Geometry check sheet. Reference: the model listing, model coordinates, mm. Give positions to 0.01 mm unless a question says otherwise; leave off trailing zeros. Order: outer loops, then holes, each group sorted by start corner. A loop starts at its lowest first (then second) coordinate and runs counter-clockwise, first axis right, second up. Notation, with made-up numbers: M -36.75,87.5 L 1.25,87.5 A19 ccw 1.25,109.5 Z; hole C -30.5,30.5 d11. An arc over 180 degrees is marked long. Use CSV: the item, a comma, the result in double quotes. Start each with the question number.
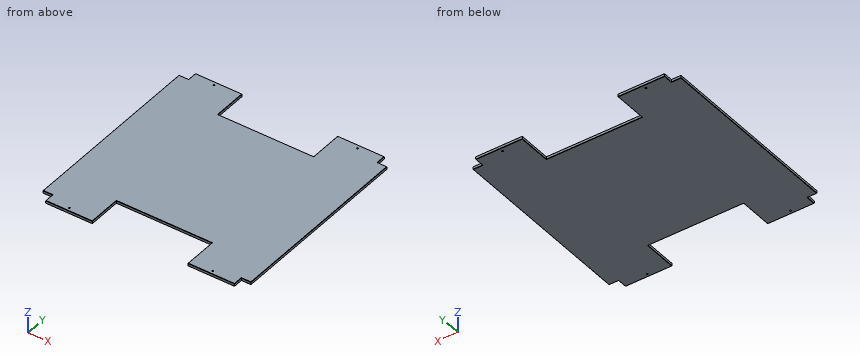
Autodesk Inventor part; units mm, degrees
ref_plane "YZ Plane" through (0, 0, 0) normal (1, 0, 0) x (0, 1, 0)
ref_plane "XZ Plane" through (0, 0, 0) normal (0, 1, 0) x (-1, 0, 0)
ref_plane "XY Plane" through (0, 0, 0) normal (0, 0, 1) x (1, 0, 0)
sketch "Skizze1" plane through (0, 0, 0) normal (0, 0, 1) x (1, 0, 0)
  line L0 (0, 0) -> (0, 395)
  line L1 (0, 395) -> (-20, 395)
  line L2 (-20, 395) -> (-20, 415)
  line L3 (-20, 415) -> (-117.5, 415)
  line L4 (-117.5, 415) -> (-117.5, 345)
  line L5 (-117.5, 345) -> (-317.5, 345)
  line L6 (-317.5, 345) -> (-317.5, 415)
  line L7 (-317.5, 415) -> (-415, 415)
  line L8 (-415, 415) -> (-415, 395)
  line L9 (-415, 395) -> (-435, 395)
  line L10 (-435, 395) -> (-435, 0)
  line L11 (-435, 0) -> (-415, 0)
  line L12 (-415, 0) -> (-415, -20)
  line L13 (-415, 0) -> (-395, 0) construction
  line L14 (-415, -20) -> (-317.5, -20)
  line L15 (-317.5, -20) -> (-317.5, 50)
  line L16 (-317.5, 50) -> (-117.5, 50)
  line L17 (-117.5, 50) -> (-117.5, -20)
  line L18 (-117.5, -20) -> (-20, -20)
  line L19 (-20, -20) -> (-20, 0)
  line L20 (-20, 0) -> (0, 0)
  dimension "d0" = 395
  dimension "d1" = 20
  dimension "d2" = 20
  dimension "d3" = 97.5
  dimension "d4" = 90
  dimension "d5" = 70
  dimension "d6" = 90
  dimension "d7" = 200
  dimension "d8" = 70
  dimension "d9" = 90
  dimension "d10" = 97.5
  dimension "d11" = 20
  dimension "d12" = 90
  dimension "d13" = 20
  dimension "d14" = 90
  dimension "d15" = 395
  dimension "d16" = 90
  dimension "d17" = 20
  dimension "d18" = 20
  dimension "d19" = 90
  dimension "d20" = 70
  dimension "d21" = 90
extrude "Extrusion1" add sketch "Skizze1" along normal blind 6
chamfer "Fase1" distance 0.5 angle 45 40 edges at (0, 197.5, 6) (-10, 0, 6) (-20, -10, 6) (-68.75, -20, 6) (-117.5, 15, 6) (-217.5, 50, 6) (-317.5, 15, 6) (-366.25, -20, 6) (-415, -10, 6) (-425, 0, 6) (-435, 197.5, 6) (-425, 395, 6) (-366.25, 415, 6) (-415, 405, 6) (-317.5, 380, 6) (-217.5, 345, 6) (-117.5, 380, 6) (-68.75, 415, 6) (-20, 405, 6) (-10, 395, 6) (-425, 0, 0) (-415, -10, 0) (-435, 197.5, 0) (-366.25, -20, 0) (-217.5, 50, 0) (-317.5, 15, 0) (-117.5, 15, 0) (-68.75, -20, 0) (-20, -10, 0) (-10, 0, 0) (0, 197.5, 0) (-10, 395, 0) (-20, 405, 0) (-68.75, 415, 0) (-117.5, 380, 0) (-217.5, 345, 0) (-317.5, 380, 0) (-425, 395, 0) (-415, 405, 0) (-366.25, 415, 0)
sketch "Skizze2" plane through (0, 0, 6) normal (0, 0, 1) x (1, 0, 0)
  circle A0 centre (-70.5, 407) radius 1.6
  line L0 (-117, 414.5) -> (-20.5, 414.5)
  line L1 (-20.5, 414.5) -> (-20.5, 394.5)
  circle A1 centre (-370.5, 407) radius 1.6
  circle A2 centre (-70.5, -13) radius 1.6
  circle A3 centre (-370.5, -13) radius 1.6
  point P0 (0, 0)
  dimension "d27" = 3.2
  dimension "d28" = 7.5
  dimension "d29" = 50
  dimension "d32" = 300
  dimension "d35" = 420
extrude "Extrusion2" cut sketch "Skizze2" against normal through all
properties part number "middle plate" material "Birke"
(1) Sectioned sample at C-C on x = -270. Record the cut outline in (y, z).
(2) Sectioned sample at A-A on z = 1.75. Record the cut outline in (x, y), then the cut area to 3 significant figures.
(3) Go/stop test with flat-tipped pins: P1, Ø3.5, axis at x = -70.5, y = -13, coming from the -Z side; P2, Ø2.5, axis at y = 408.5, z = 3.5, coming from the -X side; P3, Ø2.5, axis at x = -10, z = 3, coming from the -Y side; P4, Ø1.5, axis at x = -5.5, z = 3, coming from the +Y side. Record where each tip stops, or that it passes through.
(4) Sectioned sample at B-B on y = 19.5. Record the cut outline in (x, z), then the cut area to 3 significant figures.
(5) Thickness scan on line 1 (X direction, y = 407, z = 3.6); line 2 (Y direction, x = -70.5, z = 2.3); line 3 (X direction, y = 14, z = 3.5). Record the ranges inside material, lowest first.
Responses:
1,outline,"M 50,0.5 L 50.5,0 L 344.5,0 L 345,0.5 L 345,5.5 L 344.5,6 L 50.5,6 L 50,5.5 Z"
2,outline,"M -435,0 L -415,0 L -415,-20 L -317.5,-20 L -317.5,50 L -117.5,50 L -117.5,-20 L -20,-20 L -20,0 L 0,0 L 0,395 L -20,395 L -20,415 L -117.5,415 L -117.5,345 L -317.5,345 L -317.5,415 L -415,415 L -415,395 L -435,395 Z; hole C -370.5,-13 d3.2; hole C -370.5,407 d3.2; hole C -70.5,-13 d3.2; hole C -70.5,407 d3.2"
2,area,"160,000 mm2"
3,P1,"z = 0"
3,P2,"x = -415"
3,P3,"y = 0"
3,P4,"y = 395"
4,outline,"M -435,0.5 L -434.5,0 L -318,0 L -317.5,0.5 L -317.5,5.5 L -318,6 L -434.5,6 L -435,5.5 Z; M -117.5,0.5 L -117,0 L -0.5,0 L 0,0.5 L 0,5.5 L -0.5,6 L -117,6 L -117.5,5.5 Z"
4,area,"1,410 mm2"
5,line 1,"-415 to -372.1, -368.9 to -317.5, -117.5 to -72.1, -68.9 to -20"
5,line 2,"-20 to -14.6, -11.4 to 405.4, 408.6 to 415"
5,line 3,"-435 to -317.5, -117.5 to 0"
